Study the drawing (mm; zero at the part's minimum x, y, z) and answer. Give positions to 0.01 mm unless a question says otherwise; leave off trailing zeros. Order: outer loops, then holes, each group sorted by start corner. A loop starts at its lowest first (then second) coordinate and runs counter-clockwise, first axis right, second up.
Item 1: Given pin 1 Ø4.5 at (x, z) = (40, 60) entering from -Y, flat-ended and moving along its own axis, determine where the tip first touches the part or whether it passes through.
Item 2: A cutting plane is placed at C-C (z = 54). Write down the section's boundary in (x, y).
Item 3: A cutting plane is placed at B-B (y = 4.25). Write down the section's boundary in (x, z), plus the area to 3 significant figures.
Item 4: Find the intervals of material crossed by line 1 along Z through (x, y) = (20, 0.25); line 2 along X through (y, z) = (0.35, 40); line 3 along X through (y, z) = (12, 60), in increasing order.
Item 5: A cutting plane is placed at D-D (x = 12.5). Write down the section's boundary in (y, z), plus the area to 3 significant figures.
Item 6: A cutting plane is placed at A-A (x = 40). Write down the section's boundary in (y, z), plus the area to 3 significant figures.
Item 7: The mould has two halves that part along X. Classify the marked faces 1, 2, 3 and 4: +X half, -X half, draft (parallel to the pull), parting line (faces both ways), or undercut.
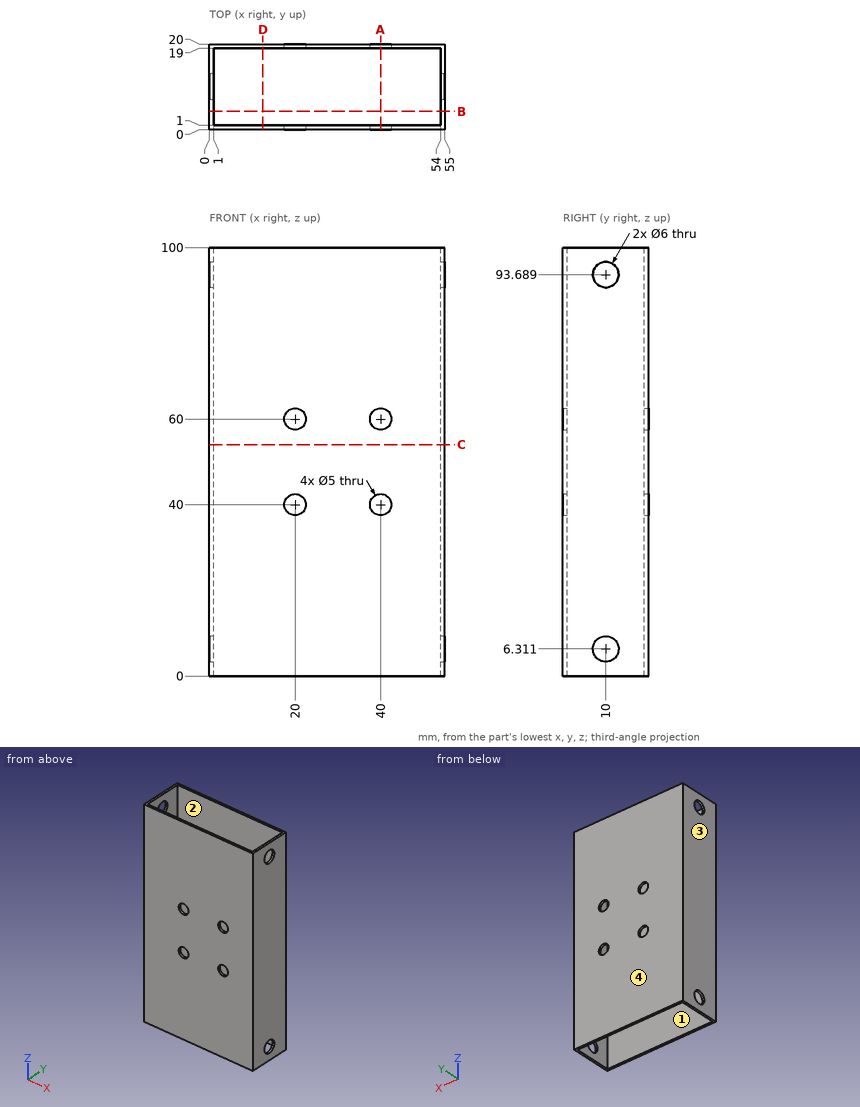
Response values:
1. pin 1: passes through
2. outline: (0, 0) - (55, 0) - (55, 20) - (0, 20) - close; hole (1, 1) - (54, 1) - (54, 19) - (1, 19) - close
3. outline: (0, 0) - (1, 0) - (1, 100) - (0, 100) - close; (54, 0) - (55, 0) - (55, 100) - (54, 100) - close
3. area: 200 mm2
4. line 1: z = 0 to 37.5, 42.5 to 57.5, 62.5 to 100
4. line 2: x = 0 to 17.5, 22.5 to 37.5, 42.5 to 55
4. line 3: x = 0 to 1, 54 to 55
5. outline: (0, 0) - (1, 0) - (1, 100) - (0, 100) - close; (19, 0) - (20, 0) - (20, 100) - (19, 100) - close
5. area: 200 mm2
6. outline: (0, 0) - (1, 0) - (1, 37.5) - (0, 37.5) - close; (0, 42.5) - (1, 42.5) - (1, 57.5) - (0, 57.5) - close; (0, 62.5) - (1, 62.5) - (1, 100) - (0, 100) - close; (19, 0) - (20, 0) - (20, 37.5) - (19, 37.5) - close; (19, 42.5) - (20, 42.5) - (20, 57.5) - (19, 57.5) - close; (19, 62.5) - (20, 62.5) - (20, 100) - (19, 100) - close
6. area: 180 mm2
7. face 1: undercut
7. face 2: undercut
7. face 3: -X half
7. face 4: draft
